```python
from build123d import *

# Parameters (mm, degrees)
F0_R     = 11
F0_R_2   = 9.5
F0_R_3   = 4
F0_W     = 1.3
F0_H     = 2
F1_DEPTH = 2
F2_DEPTH = 5
F3_DEPTH = 10
F4_SIZE2 = 2
F4_SIZE  = 7


with BuildPart() as f1:
    # F0 (on Top) → F1 (new body)
    with BuildSketch(Plane.XY):
        Circle(F0_R)
        Circle(F0_R_2, mode=Mode.SUBTRACT)
        Circle(F0_R_2)
        Circle(F0_R_3, mode=Mode.SUBTRACT)
        Circle(F0_R_3)
        Rectangle(F0_W, F0_H, mode=Mode.SUBTRACT)
        Rectangle(F0_W, F0_H)
    extrude(amount=-F1_DEPTH)

    # F0 (on Top) → F2 (join)
    with BuildSketch(Plane.XY):
        Circle(F0_R_2)
        Circle(F0_R_3, mode=Mode.SUBTRACT)
        Circle(F0_R_3)
        Rectangle(F0_W, F0_H, mode=Mode.SUBTRACT)
        Rectangle(F0_W, F0_H)
    extrude(amount=F2_DEPTH)

    # F0 (on Top) → F3 (join)
    with BuildSketch(Plane.XY):
        Circle(F0_R_3)
        Rectangle(F0_W, F0_H, mode=Mode.SUBTRACT)
    extrude(amount=-F3_DEPTH)

    # F4
    f4_edges = [f1.edges().sort_by_distance(p)[0] for p in [
        (-4, 0, -10),
    ]]
    chamfer(f4_edges, length=F4_SIZE, length2=F4_SIZE2)


solid = f1.part
```
The model under review builds one solid part; all positions refer to its coordinate system, in mm. A direction names the side the tool comes from. Give positions to 0.01 mm unless a question says otherwise; leave off trailing zeros. Write each loop counter-clockwise with the first axis right and the second up, starting at its lowest first coordinate (ties: lowest second). Pieces come first, ordered by that corner, then holes. Notation, with made-up numbers: M 28.25,65 L 36.25,65 A20 cw 36.25,73 Z; hole C -16,87.5 d2. An arc over 180 degrees is marked long. Write item = value, one per line. Start each with the question number.
Q1. For line 1 (Z direction, x = -5.75, y = -5.25); line 2 (Y direction, x = 5, z = 4); line 3 (Y direction, x = 0.75, z = 3.25), list the stretches that pass through material, from the lowest coordinate up.
Q2. We need section C-C (x = 0). State the section outline as (y, z) points, plus the area to 3 significant figures.
Q3. We need section D-D (z = 4.25). State the section outline as (x, y) points, plus the area to 3 significant figures.
Q4. Clearance check with flat-ended pins moving along their axes: pin 1 (2 mm diameter, centred on x = -7.5, y = 8, fed in from +Z); pin 2 (8 mm diameter, centred on y = -5, z = -2.5, fed in from +X); pin 3 (3 mm diameter, centred on y = -6.5, z = -6.5, fed in from +X); pin 4 (1 mm diameter, centred on x = -0.5, z = -7, fed in from +Y). State where each tip first meets the part, or that it passes through.
Q5. Mouldability with a two-part tool opening along X and no side actions: class faces 4 (the face through (-0.867, -3.905, -2.493)), 5 (the face through (0, 0, -2)), 6 (the face through (-10, 0, 0)) as released by +X, released by -X, zero draft, split by the parting line, or undercut.
Q6. We need section B-B (y = 0). State the section outline as (x, z) points, plus the area to 3 significant figures.
Q7. We need section A-A (z = -8.25). State the section outline as (x, y) points, plus the area to 3 significant figures.
Q8. Machinability: for faces 1 (the face through (0, -1, -6)), 2 (the face through (4.38, -8.43, 2.46)), 3 (the face through (1, 0, -10)), which of the approach directions +Z, -Z, +X, -X, +Y, -Y give a long, thin tool a straight path to every point of the face, cutting with its end or side? Answer none if there is none.
Result set:
q1.line_1 = -2 to 5
q1.line_2 = -8.08 to 8.08
q1.line_3 = -9.47 to 9.47
q2.outline = M -11,-2 L -4,-2 L -4,-3 L -2,-10 L -1,-10 L -1,-2 L 1,-2 L 1,-10 L 2,-10 L 4,-3 L 4,-2 L 11,-2 L 11,0 L 9.5,0 L 9.5,5 L -9.5,5 L -9.5,0 L -11,0 Z
q2.area = 173 mm2
q3.outline = C 0,0 d19
q3.area = 284 mm2
q4.pin_1 = 0
q4.pin_2 = 10.95
q4.pin_3 = through
q4.pin_4 = 2.97
q5.face_4 = split by the parting line
q5.face_5 = undercut
q5.face_6 = zero draft
q6.outline = M -11,-2 L -4,-2 L -4,-3 L -2,-10 L -0.65,-10 L -0.65,-2 L 0.65,-2 L 0.65,-10 L 2,-10 L 4,-3 L 4,-2 L 11,-2 L 11,0 L 9.5,0 L 9.5,5 L -9.5,5 L -9.5,0 L -11,0 Z
q6.area = 179 mm2
q7.outline = C 0,0 d5; hole M -0.65,-1 L 0.65,-1 L 0.65,1 L -0.65,1 Z
q7.area = 17.0 mm2
q8.face_1 = -Z
q8.face_2 = +Z
q8.face_3 = -Z, +X, -X, +Y, -Y
